The figure shows three views and two pictorial views of one solid part (mm, origin at its lowest corner). Answer the questions. A direction names the side the tool comes from. Coordinates: 2 decimals unless noted, no trailing zeros. Loops run counter-clockwise (first coordinate to the right, second up) from the corner with the lowest first, then second, coordinate; pieces in that order, holes last. Notation, with made-up numbers: (38, 12.5) - (52, 12.5) arc R12 cw to (52, 19.5) - close; hole circle Ø11 at (-2.5, -22.5). An arc over 180 degrees is marked (long way). One line per question, with ' | ' between items.
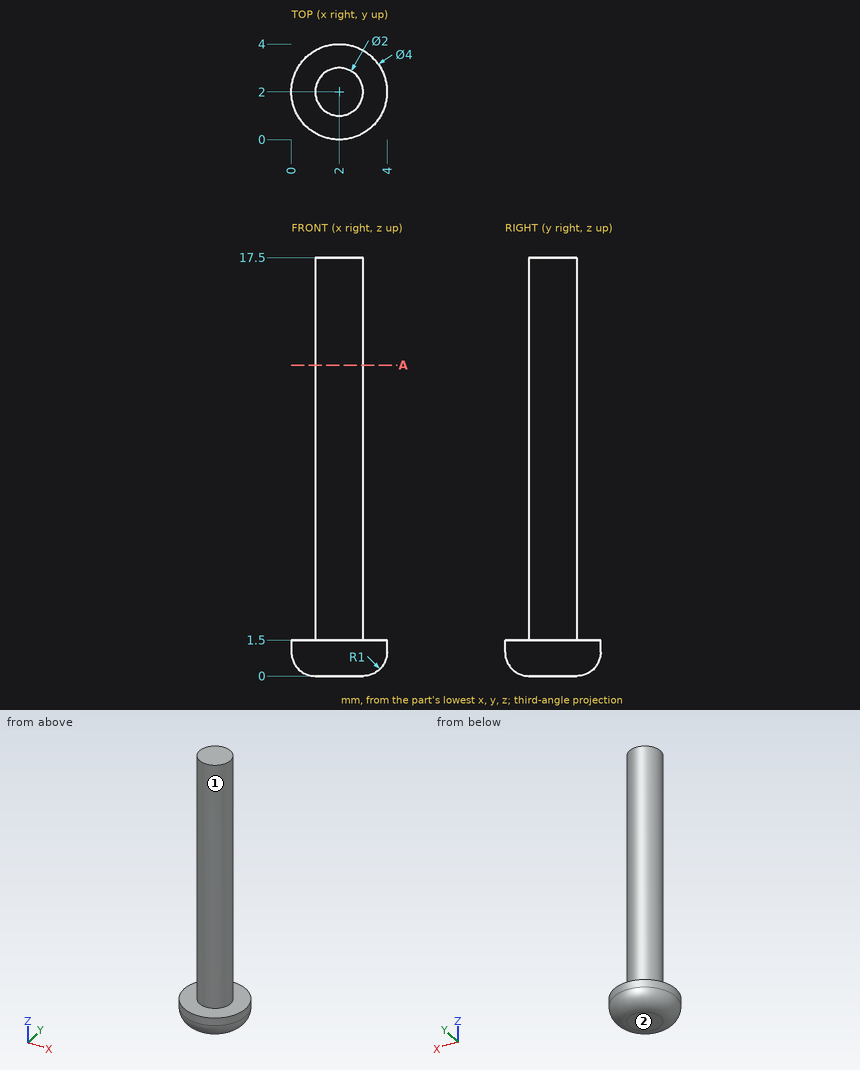
Item 1: Which of the six approach directions +Z, -Z, +X, -X, +Y, -Y give full straight-line access (tool end or side, diameter ignored) to the marked faces 1 and 2?
Taken from the geometry:
face 1: +Z | face 2: -Z, +X, -X, +Y, -Y
Item 2: Each of these flat-tipped pins is pushed along its axis until it touches: pin 1 Ø1.5 at (x, y) = (1.5, 3.5) entering from +Z; pin 2 Ø1 at (y, z) = (1.5, 5.5) entering from +X; pin 3 Ø1.5 at (x, z) = (1, 10.5) entering from -Y. Where does it stop, or does it pass through?
Taken from the geometry:
pin 1: stops at z = 17.5 | pin 2: stops at x = 3 | pin 3: stops at y = 1.03
Item 3: Find section A-A, the plane z = 13. Write down the section's boundary in (x, y), plus the area to 3 significant figures.
Taken from the geometry:
outline: circle Ø2 at (2, 2) | area: 3.14 mm2
Item 4: Find the intervals of material crossed by line 1 (Y direction, x = 1.95, z = 14); line 2 (X direction, y = 1.5, z = 13.5); line 3 (X direction, y = 2.55, z = 9.5), in increasing order. Write a range as [from, to].
Taken from the geometry:
line 1: y = [1, 3] | line 2: x = [1.13, 2.87] | line 3: x = [1.16, 2.84]
